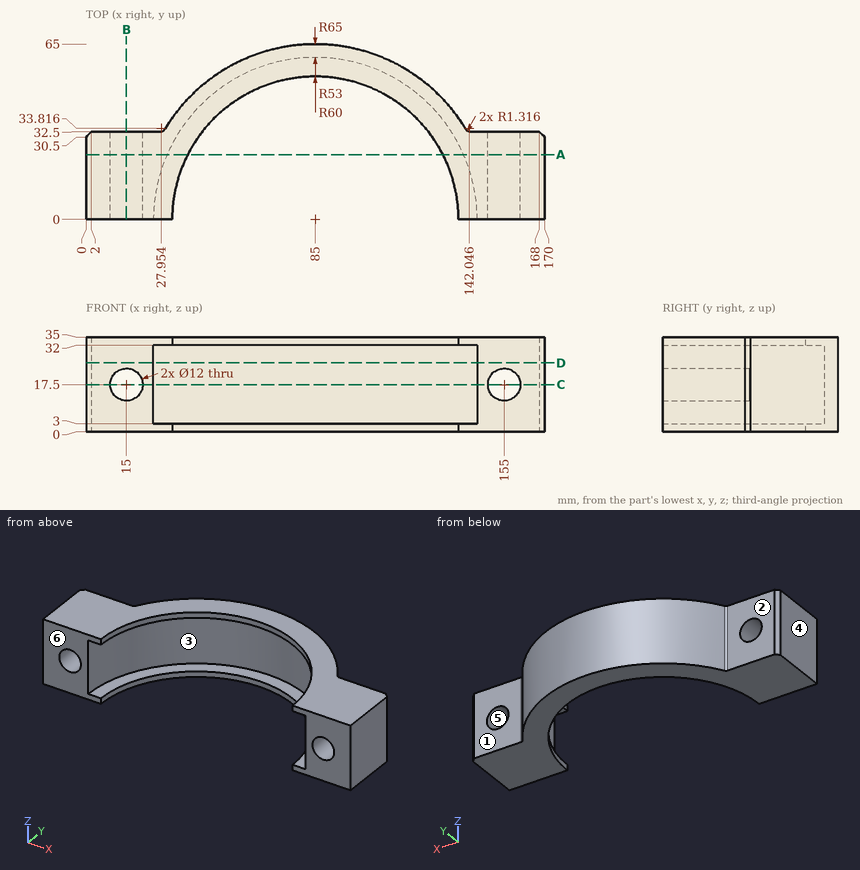
Answer from the drawing. Dimensions are ordinates in mm from the lowest x, y and z of the part. A direction names the side the tool comes from. Round coordinates to 2 decimals unless told otherwise and drop trailing zeros. Loops run counter-clockwise (first coordinate to the right, second up) from the corner with the lowest first, then second, coordinate; pieces in that order, holes last. Notation, with made-up numbers: M -13.75,1 L 0.25,1 A6 cw 0.25,8 Z; hole C -0.5,31.25 d5. An arc over 180 degrees is marked long. One line per question, with ' | ' between items. Start each with the question number.
(1) A cutting plane is placed at C-C on z = 17.5. Write down the section's boundary in (x, y) (1 decimal), plus the area to 3 significant figures.
(2) A cutting plane is placed at D-D on z = 25.5. Write down the section's boundary in (x, y) (1 decimal), plus the area to 3 significant figures.
(3) Find the intervals of material crossed by line 1 (X direction, y = 14, z = 17.5); line 2 (Z direction, x = 29.5, y = 15.5); line 3 (Z direction, x = 15, y = 9), in increasing order.
(4) For a pull along X with two mould halves and no side action, classify the marked faces 4, 5 and 6 as released by +X, released by -X, zero draft, split by the parting line, or undercut.
(5) A cutting plane is placed at B-B on x = 15. Write down the section's boundary in (y, z).
(6) A cutting plane is placed at A-A on y = 24. Write down the section's boundary in (x, z) (1 decimal).
(7) A tool of negligible diameter and unlimited length cuts with its end or side. For the marked faces 1, 2 and 3, from which of +Z, -Z, +X, -X, +Y, -Y can it reach the whole face along a straight path? Write none if from no direction.
(8) Flat-ended cylindrical pins translate along their axes: pin 1 Ø14 at (x, z) = (155, 17.5) entering from +Y; pin 2 Ø10 at (x, z) = (39.5, 11) entering from +Y; pin 3 Ø6 at (x, z) = (73, 16) entering from -Y (1 decimal). Find the tip coordinate at first contact, or state that the pin passes through.
Geometry check:
1) outline: M 0,0 L 9,0 L 9,32.5 L 2,32.5 L 0,30.5 Z; M 21,0 L 25,0 A60 cw 145,0 L 149,0 L 149,32.5 L 142,32.5 A1.3 cw 140.9,33.1 A65 ccw 29.1,33.1 A1.3 cw 28,32.5 L 21,32.5 Z; M 161,0 L 170,0 L 170,30.5 L 168,32.5 L 161,32.5 Z | area: 1,680 mm²
2) outline: M 0,0 L 25,0 A60 cw 145,0 L 170,0 L 170,30.5 L 168,32.5 L 142,32.5 A1.3 cw 140.9,33.1 A65 ccw 29.1,33.1 A1.3 cw 28,32.5 L 2,32.5 L 0,30.5 Z | area: 2,460 mm²
3) line 1: x = 0 to 9, 21 to 26.66, 143.34 to 149, 161 to 170 | line 2: z = 0 to 3, 32 to 35 | line 3: z = 0 to 11.5, 23.5 to 35
4) face 4: released by -X | face 5: undercut | face 6: zero draft
5) outline: M 0,0 L 32.5,0 L 32.5,11.5 L 0,11.5 Z; M 0,23.5 L 32.5,23.5 L 32.5,35 L 0,35 Z
6) outline: M 0,0 L 37.7,0 L 37.7,3 L 30,3 L 30,32 L 37.7,32 L 37.7,35 L 0,35 Z; M 132.3,0 L 170,0 L 170,35 L 132.3,35 L 132.3,32 L 140,32 L 140,3 L 132.3,3 Z; hole C 15,17.5 d12; hole C 155,17.5 d12
7) face 1: +Z, -Z, +X, +Y | face 2: +Z, -Z, -X, +Y | face 3: -Y
8) pin 1: stops at y = 32.5 | pin 2: stops at y = 50.84 | pin 3: stops at y = 58.1
